Model file for the job. Use its own axes, mm. Round coordinates to 2 decimals unless told otherwise and drop trailing zeros. Loops run counter-clockwise (first coordinate to the right, second up) from the corner with the lowest first, then second, coordinate; pieces in that order, holes last. Notation, with made-up numbers: (-3.75, 50.25) -> (55.25, 50.25) arc R14 cw to (55.25, 61.25) -> close; hole circle Ø11 at (55.5, 16). An arc over 180 degrees is marked (long way). Use a Markdown table: item, result. Add a question column.
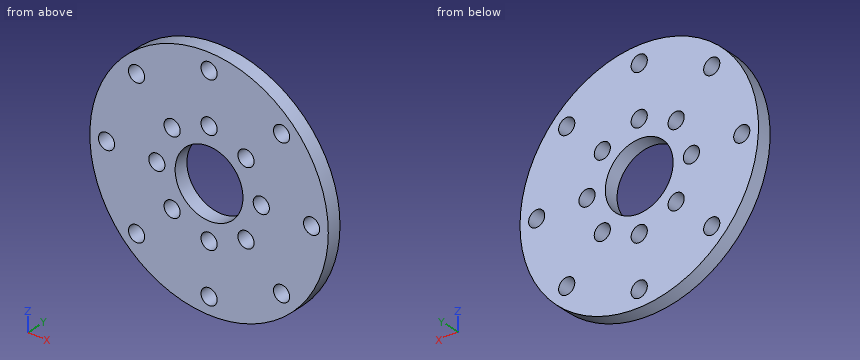
```python
from build123d import *

# Parameters (mm, degrees)
CROQUIS1_R              = 22.15
CROQUIS1_R_2            = 6.3
CROQUIS1_R_3            = 1.5
SALIENTE_EXTRUIR1_DEPTH = 2.7


with BuildPart() as part:
    # Croquis1 → Saliente-Extruir1 (new body)
    with BuildSketch(Plane(origin=(0, 0, 0), x_dir=(1, 0, 0), z_dir=(0, 1, 0))):
        Circle(CROQUIS1_R)
        Circle(CROQUIS1_R_2, mode=Mode.SUBTRACT)
        with Locations((0, 19.05)):
            Circle(CROQUIS1_R_3, mode=Mode.SUBTRACT)
        with Locations((13.470384182, 13.470384182)):
            Circle(CROQUIS1_R_3, mode=Mode.SUBTRACT)
        with Locations((19.05, 0)):
            Circle(CROQUIS1_R_3, mode=Mode.SUBTRACT)
        with Locations((13.470384182, -13.470384182)):
            Circle(CROQUIS1_R_3, mode=Mode.SUBTRACT)
        with Locations((0, -19.05)):
            Circle(CROQUIS1_R_3, mode=Mode.SUBTRACT)
        with Locations((-13.470384182, -13.470384182)):
            Circle(CROQUIS1_R_3, mode=Mode.SUBTRACT)
        with Locations((-19.05, 0)):
            Circle(CROQUIS1_R_3, mode=Mode.SUBTRACT)
        with Locations((-13.470384182, 13.470384182)):
            Circle(CROQUIS1_R_3, mode=Mode.SUBTRACT)
        with Locations((0, 9.7)):
            Circle(CROQUIS1_R_3, mode=Mode.SUBTRACT)
        with Locations((6.858935778, 6.858935778)):
            Circle(CROQUIS1_R_3, mode=Mode.SUBTRACT)
        with Locations((9.7, 0)):
            Circle(CROQUIS1_R_3, mode=Mode.SUBTRACT)
        with Locations((6.858935778, -6.858935778)):
            Circle(CROQUIS1_R_3, mode=Mode.SUBTRACT)
        with Locations((0, -9.7)):
            Circle(CROQUIS1_R_3, mode=Mode.SUBTRACT)
        with Locations((-6.858935778, -6.858935778)):
            Circle(CROQUIS1_R_3, mode=Mode.SUBTRACT)
        with Locations((-9.7, 0)):
            Circle(CROQUIS1_R_3, mode=Mode.SUBTRACT)
        with Locations((-6.858935778, 6.858935778)):
            Circle(CROQUIS1_R_3, mode=Mode.SUBTRACT)
    extrude(amount=SALIENTE_EXTRUIR1_DEPTH)


solid = part.part
```
1) Wall check: probe 1 along Z at (x, y) = (0, 1.05); probe 2 along Z at (x, y) = (-13.5, 1). Give the ranges that are in metal, low to high. Write a range as from..to.
2) Cut at D-D on x = -13. Write the cut outline in (y, z).
3) Pin check, flat tips, straight feed: pin 1 Ø4 at (x, z) = (-6.86, 6.86) entering from -Y; pin 2 Ø1.5 at (y, z) = (1, -12) entering from +X; pin 3 Ø1 at (x, y) = (-16.5, 2) entering from +Z. Stop position of each tip, or through.
4) Cut at B-B on x = 2.5. Write the cut outline in (y, z).
5) Cut at A-A on z = 0. Write the cut outline in (x, y), and give its area (3 significant figures).
6) Cut at C-C on y = 2.05. Count the separate pieces of the cut face and the enclosed holes in it, and give its area (3 significant figures).
Established:
| question | item | result |
|---|---|---|
| 1 | probe 1 | z = -22.15..-20.55, -17.55..-11.2, -8.2..-6.3, 6.3..8.2, 11.2..17.55, 20.55..22.15 |
| 1 | probe 2 | z = -17.56..-14.97, -11.97..11.97, 14.97..17.56 |
| 2 | outline | (0, -17.93) -> (2.7, -17.93) -> (2.7, -14.89) -> (0, -14.89) -> close; (0, -12.05) -> (2.7, -12.05) -> (2.7, 12.05) -> (0, 12.05) -> close; (0, 14.89) -> (2.7, 14.89) -> (2.7, 17.93) -> (0, 17.93) -> close |
| 3 | pin 1 | stops at y = 0 |
| 3 | pin 2 | stops at x = 19.08 |
| 3 | pin 3 | stops at z = 15.32 |
| 4 | outline | (0, -22.01) -> (2.7, -22.01) -> (2.7, -5.78) -> (0, -5.78) -> close; (0, 5.78) -> (2.7, 5.78) -> (2.7, 22.01) -> (0, 22.01) -> close |
| 5 | outline | (-22.15, 0) -> (-20.55, 0) -> (-20.55, 2.7) -> (-22.15, 2.7) -> close; (-17.55, 0) -> (-11.2, 0) -> (-11.2, 2.7) -> (-17.55, 2.7) -> close; (-8.2, 0) -> (-6.3, 0) -> (-6.3, 2.7) -> (-8.2, 2.7) -> close; (6.3, 0) -> (8.2, 0) -> (8.2, 2.7) -> (6.3, 2.7) -> close; (11.2, 0) -> (17.55, 0) -> (17.55, 2.7) -> (11.2, 2.7) -> close; (20.55, 0) -> (22.15, 0) -> (22.15, 2.7) -> (20.55, 2.7) -> close |
| 5 | area | 53.2 mm^2 |
| 6 | separate pieces | 1 |
| 6 | enclosed holes | 17 |
| 6 | area | 1,300 mm^2 |
